from build123d import *

# Parameters (mm, degrees)
F1_DEPTH = 75
F2_R     = 5
F3_DEPTH = 25
F5_DEPTH = 25
F7_R     = 10
F8_DEPTH = 10


with BuildPart() as f1:
    # F0 (on Front) → F1 (new body)
    with BuildSketch(Plane.XZ):
        with BuildLine():
            Line((-50, 0), (0, 0))
            ThreePointArc((0, 0), (17.67767, 7.32233), (25, 25))
            Line((25, 25), (25, 35))
            Line((25, 35), (70, 35))
            Line((70, 35), (70, 50))
            Line((70, 50), (0, 50))
            ThreePointArc((0, 50), (-17.67767, 42.67767), (-25, 25))
            Line((-25, 25), (-25, 15))
            Line((-25, 15), (-40, 15))
            Line((-40, 15), (-40, 75))
            Line((-40, 75), (-50, 75))
            Line((-50, 75), (-50, 0))
        make_face()
        with BuildLine():
            ThreePointArc((0, 10), (-10.606602, 35.606602), (15, 25))
            ThreePointArc((15, 25), (10.606602, 14.393398), (0, 10))
        make_face(mode=Mode.SUBTRACT)
    extrude(amount=F1_DEPTH)

    # F2 (on face) → F3 (cut)
    with BuildSketch(Plane.XY.offset(50)):
        with Locations((55, -20)):
            Circle(F2_R)
        with Locations((55, -55)):
            Circle(F2_R)
    extrude(amount=-F3_DEPTH, mode=Mode.SUBTRACT)

    # F4 (on face) → F5 (cut)
    with BuildSketch(Plane(origin=(-50, 0, 0), x_dir=(0, -1, 0), z_dir=(-1, 0, 0))):
        Polygon((0, 60), (15, 75), (0, 75), align=None)
        Polygon((75, 75), (60, 75), (75, 60), align=None)
    extrude(amount=-F5_DEPTH, mode=Mode.SUBTRACT)

    # F7 (on face) → F8 (cut)
    with BuildSketch(Plane.YZ.offset(-40)):
        with Locations((-38.184846, 37.546992)):
            Circle(F7_R)
    extrude(amount=-F8_DEPTH, mode=Mode.SUBTRACT)


solid = f1.part
Model file for the job. Use its own axes, mm. A direction names the side the tool comes from. Round coordinates to 2 decimals unless told otherwise and drop trailing zeros. Order: outer loops, then holes, each group sorted by start corner. A loop starts at its lowest first (then second) coordinate and runs counter-clockwise, first axis right, second up.
(1) Band-saw the part on A-A (y = -41). List the corners of the cut face in (x, z).
(2) Pin check, flat tips, straight feed: pin 1 (6 mm diameter, centred on y = -31.5, z = 58, fed in from +X); pin 2 (16 mm diameter, centred on x = 55, y = -55, fed in from +Z); pin 3 (4.5 mm diameter, centred on x = -35, y = -32, fed in from +Z); pin 4 (12 mm diameter, centred on x = 54.5, z = 57.5, fed in from -Y). Stop position of each tip, or through.
(3) Band-saw the part on D-D (y = -13). List the corners of the cut face in (x, z).
(4) Band-saw the part on B-B (z = 43). List the corners of the cut face in (x, y), then the cut area to 3 significant figures.
(5) 3-axis set-ups, long thin cutter, end or side, ignore diameter. For faces 5 (the face through (35, -37, 50)), 6 (the face through (47, -37, 35)), 7 (the face through (-25, -37, 20)): which of +Z, -Z, +X, -X, +Y, -Y reach the whole face in a straight line?
(6) Band-saw the part on C-C (x = 55). List the corners of the cut face in (y, z).
(7) Pull direction Y, two halves, no side cores. Call faces 1 (the face through (54.349, -50.043, 42.605)), 2 (the face through (53.92, -24.88, 42.6)), 3 (the face through (-18, -75, 30)), 4 (the face through (17.482, -36.975, 7.129)): released by +Y, released by -Y, zero draft, split by the parting line, or undercut.
(8) Drill centre lines: line 1 (X direction, y = -46, z = 25.5) (3 decimals); line 2 (Y direction, x = 55, z = 41.5); line 3 (X direction, y = -48, z = 27). Where is each one in solid material? Low to high.
Verdict:
1. outline: (-50, 0) - (0, 0) arc R25 ccw to (25, 25) - (25, 35) - (70, 35) - (70, 50) - (0, 50) arc R25 ccw to (-25, 25) - (-25, 15) - (-40, 15) - (-40, 27.95) - (-50, 27.95) - close; (-50, 47.14) - (-40, 47.14) - (-40, 75) - (-50, 75) - close; hole (0, 10) arc R15 ccw to (15, 25) arc R15 ccw (long way) to start
2. pin 1: stops at x = -40
2. pin 2: stops at z = 50
2. pin 3: stops at z = 15
2. pin 4: passes through
3. outline: (-50, 0) - (0, 0) arc R25 ccw to (25, 25) - (25, 35) - (70, 35) - (70, 50) - (0, 50) arc R25 ccw to (-25, 25) - (-25, 15) - (-40, 15) - (-40, 73) - (-50, 73) - close; hole (0, 10) arc R15 ccw to (15, 25) arc R15 ccw (long way) to start
4. outline: (-50, -75) - (-40, -75) - (-40, -46.57) - (-50, -46.57) - close; (-50, -29.8) - (-40, -29.8) - (-40, 0) - (-50, 0) - close; (-17.35, -75) - (70, -75) - (70, 0) - (-17.35, 0) - close; hole circle Ø10 at (55, -55); hole circle Ø10 at (55, -20)
4. area: 6,980 mm2
5. face 5: +Z, +X, +Y, -Y
5. face 6: -Z, +X, +Y, -Y
5. face 7: +Z, +Y, -Y
6. outline: (-75, 35) - (-60, 35) - (-60, 50) - (-75, 50) - close; (-50, 35) - (-25, 35) - (-25, 50) - (-50, 50) - close; (-15, 35) - (0, 35) - (0, 50) - (-15, 50) - close
7. face 1: undercut
7. face 2: undercut
7. face 3: released by -Y
7. face 4: zero draft
8. line 1: x = -50 to -40, -24.995 to -14.992, 14.992 to 25
8. line 2: y = -75 to -60, -50 to -25, -15 to 0
8. line 3: x = -50 to -40, -24.92 to -14.87, 14.87 to 25
